Source: CAD feature listing. Evaluate the final solid. Frame: model axes, mm. Give positions to 0.01 mm unless a question says otherwise; leave off trailing zeros. Loops run counter-clockwise (first coordinate to the right, second up) from the corner with the lowest first, then second, coordinate; pieces in that order, holes last. Notation, with made-up numbers: (-2.75, 20.25) -> (46.25, 20.25) arc R24 cw to (46.25, 49.25) -> close; hole circle Ø4 at (-27.75, 42.5). An arc over 180 degrees is marked (long way). Put each result on its own line as item: value.
```python
from build123d import *

# Parameters (mm, degrees)
SKETCH1_W           = 91
SKETCH1_H           = 91
SKETCH1_R           = 3.175
SKETCH1_R_2         = 1.524
BOSS_EXTRUDE1_DEPTH = 1.5


with BuildPart() as part:
    # Sketch1 → Boss-Extrude1 (new body)
    with BuildSketch(Plane(origin=(0, 0, 0), x_dir=(1, 0, 0), z_dir=(0, 1, 0))):
        Rectangle(SKETCH1_W, SKETCH1_H)
        with Locations((-40.5, -40.5)):
            Circle(SKETCH1_R, mode=Mode.SUBTRACT)
        with Locations((40.5, -40.5)):
            Circle(SKETCH1_R, mode=Mode.SUBTRACT)
        with Locations((40.5, 40.5)):
            Circle(SKETCH1_R, mode=Mode.SUBTRACT)
        with Locations((-40.5, 40.5)):
            Circle(SKETCH1_R, mode=Mode.SUBTRACT)
        with Locations((-40.5, -40.5)):
            Circle(SKETCH1_R)
        with Locations((-40.5, -40.5)):
            Circle(SKETCH1_R_2, mode=Mode.SUBTRACT)
        with Locations((-40.5, 40.5)):
            Circle(SKETCH1_R)
        with Locations((-40.5, 40.5)):
            Circle(SKETCH1_R_2, mode=Mode.SUBTRACT)
        with Locations((40.5, 40.5)):
            Circle(SKETCH1_R)
        with Locations((40.5, 40.5)):
            Circle(SKETCH1_R_2, mode=Mode.SUBTRACT)
        with Locations((40.5, -40.5)):
            Circle(SKETCH1_R)
        with Locations((40.5, -40.5)):
            Circle(SKETCH1_R_2, mode=Mode.SUBTRACT)
    extrude(amount=BOSS_EXTRUDE1_DEPTH)


solid = part.part
```
(1) Section B-B on z = -40.5. Return loops of the section in (x, y).
Calculated:
outline: (-45.5, 0) -> (-42.02, 0) -> (-42.02, 1.5) -> (-45.5, 1.5) -> close; (-38.98, 0) -> (38.98, 0) -> (38.98, 1.5) -> (-38.98, 1.5) -> close; (42.02, 0) -> (45.5, 0) -> (45.5, 1.5) -> (42.02, 1.5) -> close
(2) Section A-A on x = -40.5. Return loops of the section in (y, z).
Calculated:
outline: (0, -45.5) -> (1.5, -45.5) -> (1.5, -42.02) -> (0, -42.02) -> close; (0, -38.98) -> (1.5, -38.98) -> (1.5, 38.98) -> (0, 38.98) -> close; (0, 42.02) -> (1.5, 42.02) -> (1.5, 45.5) -> (0, 45.5) -> close
(3) Line query: probe 1 along Z at (x, y) = (40.5, 0.4); probe 2 along X at (y, z) = (0.9, 40). Output: solid intervals per line, ascending. Write a range as from..to.
Calculated:
probe 1: z = -45.5..-42.02, -38.98..38.98, 42.02..45.5
probe 2: x = -45.5..-41.94, -39.06..39.06, 41.94..45.5
(4) Draft query along X for faces 1 (the cylindrical face through (-41.709, 0.74, 41.427)), 2 (the flat face through (-1, 0, -1)), 3 (the cylindrical face through (-41.709, 0.74, -39.573)). Return one class per face: released by +X, released by -X, zero draft, split by the parting line, or undercut.
Calculated:
face 1: undercut
face 2: zero draft
face 3: undercut
